```python
from build123d import *

# Parameters (mm, degrees)
F0_W      = 88
F0_H      = 15
F1_DEPTH  = 14
F3_DEPTH  = 24.5
F4_W      = 113
F4_H      = 15
F5_DEPTH  = 12
F6_W      = 34.5
F6_H      = 5
F7_DEPTH  = 25
F8_R      = 1.5
F9_DEPTH  = 25
F10_W     = 17.581136
F10_H     = 6
F11_DEPTH = 3
F12_R     = 2
F13_R     = 2
F14_DEPTH = 25


with BuildPart() as f1:
    # F0 (on Front) → F1 (new body)
    with BuildSketch(Plane.XZ):
        Rectangle(F0_W, F0_H)
    extrude(amount=F1_DEPTH)

    # F2 (on face) → F3 (cut)
    with BuildSketch(Plane.XZ.offset(14)):
        Polygon((-33.5, 1.5), (-33.5, -7.5), (44, -7.5), (44, 7.5), (18.5, 7.5), (18.5, 1.5), align=None)
    extrude(amount=-F3_DEPTH, mode=Mode.SUBTRACT)

    # F4 (on face) → F5 (join)
    with BuildSketch(Plane.XZ.offset(14)):
        with Locations((12.5, 0)):
            Rectangle(F4_W, F4_H)
    extrude(amount=-F5_DEPTH)

    # F6 (on face) → F7 (cut)
    with BuildSketch(Plane(origin=(0, -2, 0), x_dir=(-1, 0, 0), z_dir=(0, 1, 0))):
        with Locations((-47.75, -3)):
            Rectangle(F6_W, F6_H)
    extrude(amount=-F7_DEPTH, mode=Mode.SUBTRACT)

    # F8 (on face) → F9 (cut)
    with BuildSketch(Plane.XZ.offset(14)):
        with Locations((17, -3)):
            Circle(F8_R)
    extrude(amount=-F9_DEPTH, mode=Mode.SUBTRACT)

    # F10 (on face) → F11 (cut)
    with BuildSketch(Plane(origin=(0, -2, 0), x_dir=(-1, 0, 0), z_dir=(0, 1, 0))):
        with Locations((-17, -3)):
            Rectangle(F10_W, F10_H)
    extrude(amount=-F11_DEPTH, mode=Mode.SUBTRACT)

    # F12
    f12_edges = [f1.edges().sort_by_distance(p)[0] for p in [
        (8.209432, -3.5, 0),
        (8.209432, -3.5, -6),
        (25.790568, -3.5, 0),
        (25.790568, -3.5, -6),
    ]]
    fillet(f12_edges, radius=F12_R)

    # F13 (on face) → F14 (cut)
    with BuildSketch(Plane.XZ.offset(14)):
        with Locations((-38, 0)):
            Circle(F13_R)
    extrude(amount=-F14_DEPTH, mode=Mode.SUBTRACT)


solid = f1.part
```
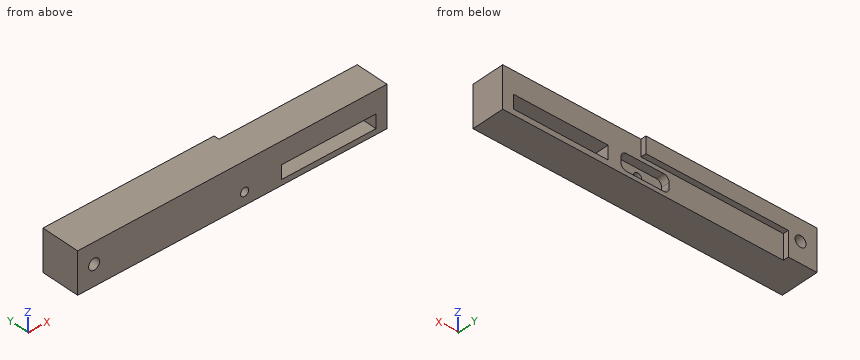
Build history of the part. All positions in model axes, mm. Coordinates: 2 decimals unless noted, no trailing zeros. Write each loop counter-clockwise with the first axis right and the second up, starting at its lowest first coordinate (ties: lowest second). Pieces come first, ordered by that corner, then holes.
1. Band-saw the part on D-D, the plane x = -15. Give the cut face in (y, z).
Answer block:
outline: (-14, -7.5) - (-2, -7.5) - (-2, 1.5) - (0, 1.5) - (0, 7.5) - (-14, 7.5) - close
2. Band-saw the part on A-A, the plane x = -38. Give the cut face in (y, z).
Answer block:
outline: (-14, -7.5) - (0, -7.5) - (0, -2) - (-14, -2) - close; (-14, 2) - (0, 2) - (0, 7.5) - (-14, 7.5) - close
3. Band-saw the part on C-C, the plane z = -3. Give the cut face in (x, y).
Answer block:
outline: (-44, -14) - (15.5, -14) - (15.5, -5) - (8.21, -5) - (8.21, -2) - (-33.5, -2) - (-33.5, 0) - (-44, 0) - close; (18.5, -14) - (30.5, -14) - (30.5, -2) - (25.79, -2) - (25.79, -5) - (18.5, -5) - close; (65, -14) - (69, -14) - (69, -2) - (65, -2) - close
4. Drop flat-ended pins along their axis: pin 1 (6.5 mm diameter, centred on x = 14.5, z = -2, fed in from +Y); pin 2 (1 mm diameter, centred on y = -1, z = 5, fed in from +X); pin 3 (4.5 mm diameter, centred on x = 20, z = -3, fed in from +Y); pin 4 (2.5 mm diameter, centred on x = 17, z = -3, fed in from +Y). Give the stop position or say it passes through.
Answer block:
pin 1: stops at y = -2
pin 2: stops at x = 18.5
pin 3: stops at y = -5
pin 4: passes through
5. Drill centre lines: probe 1 along X at (y, z) = (-11.5, -5.25); probe 2 along Z at (x, y) = (17, -10); probe 3 along Z at (x, y) = (52, -9.5). Where is each one in solid material? Low to high.
Answer block:
probe 1: x = -44 to 30.5, 65 to 69
probe 2: z = -7.5 to -4.5, -1.5 to 7.5
probe 3: z = -7.5 to -5.5, -0.5 to 7.5
6. Band-saw the part on B-B, the plane y = -6. Give the cut face in (x, z), and give its area (3 significant figures).
Answer block:
outline: (-44, -7.5) - (69, -7.5) - (69, 7.5) - (-44, 7.5) - close; hole circle Ø4 at (-38, 0); hole circle Ø3 at (17, -3); hole (30.5, -5.5) - (65, -5.5) - (65, -0.5) - (30.5, -0.5) - close
area: 1,500 mm2
